Source: CAD feature listing. Evaluate the final solid. Frame: model axes, mm. Face numbers are marked on the shaded views. A direction names the side the tool comes from. Round coordinates to 2 decimals unless told otherwise and drop trailing zeros. Loops run counter-clockwise (first coordinate to the right, second up) from the corner with the lowest first, then second, coordinate; pieces in that order, holes last. Notation, with made-up numbers: (86.25, 60) -> (124.25, 60) arc R22 ccw to (124.25, 72) -> close; hole circle Ø11 at (-13, -39). An arc over 180 degrees is marked (long way). Put each result on its own line as item: value. Start each with the question number.
1. Cut plane D-D (z = 1.5). Return the cut outline in (x, y), then the cut area to 3 significant figures.
2. Cut plane B-B (y = 6.5). Return the cut outline in (x, z).
3. Contact query for flat-ended pins moving along their axis: pin 1 (1.5 mm diameter, centred on x = -18, y = 3.5, fed in from +Z); pin 2 (5.5 mm diameter, centred on y = 12, z = 8.5, fed in from -X); pin 3 (3 mm diameter, centred on x = -7, y = 14.5, fed in from +Z); pin 4 (5 mm diameter, centred on x = -7, y = 8.5, fed in from +Z). Output: stop coordinate, or through.
4. Material intervals for L1, parallel to Y at x = -1.25, z = 17.75; L2, parallel to Z at x = -3.5, y = 13.75; L3, parallel to Z at x = -16.5, y = 12, sorted ascending.
5. Set-up query: the marked faces 1, 2, 3, 4 and 5. Return all of +Z, -Z, +X, -X, +Y, -Y with unobstructed straight access to the full face (end or side cutting, diameter ignored); none if empty.
6. Cut plane C-C (z = 3.5). Return the cut outline in (x, y).
7. Cut plane A-A (x = -16). Return the cut outline in (y, z), then the cut area to 4 significant figures.
```python
from build123d import *

# Parameters (mm, degrees)
BOSS_EXTRUDE1_DEPTH = 20
CUT_EXTRUDE5_DEPTH  = 30
BOSS_EXTRUDE5_DEPTH = 20
CUT_EXTRUDE9_DEPTH  = 22
CUT_EXTRUDE10_DEPTH = 22
BOSS_EXTRUDE6_DEPTH = 5
BOSS_EXTRUDE7_DEPTH = 5
BOSS_EXTRUDE8_DEPTH = 5
CUT_EXTRUDE11_DEPTH = 5


with BuildPart() as part:
    # Sketch1 → Boss-Extrude1 (new body)
    with BuildSketch(Plane(origin=(0, 0, 0), x_dir=(1, 0, 0), z_dir=(0, 1, 0))):
        Polygon((-15, 0), (0, 0), (0, -15), (-5, -15), (-5, -10), align=None)
    extrude(amount=BOSS_EXTRUDE1_DEPTH)

    # Sketch8 → Cut-Extrude5 (cut)
    with BuildSketch(Plane.ZY.offset(5)):
        Polygon((10, 20), (15, 15), (15, 20), align=None)
    extrude(amount=-CUT_EXTRUDE5_DEPTH, mode=Mode.SUBTRACT)

    # Sketch9 → Boss-Extrude5 (add)
    with BuildSketch(Plane(origin=(0, 0, 0), x_dir=(-1, 0, 0), z_dir=(0, -1, 0))):
        Polygon((15, 0), (5, -10), (5, -15), (15, -15), align=None)
    extrude(amount=-BOSS_EXTRUDE5_DEPTH)

    # 3DSketch3 → Cut-Extrude9 (cut, along a direction that is not the sketch's normal)
    with BuildSketch(Plane(origin=(-15, 20, 0), x_dir=(0.2672612419124245, -0.5345224838248489, 0.8017837257372732), z_dir=(-0.5773502691896256, 0.5773502691896258, 0.5773502691896258))):
        Polygon((0, 0), (10.690449676, 9.258200998), (17.371980724, 6.943650748), (18.708286934, 0), (13.363062096, -4.629100499), align=None)
    extrude(amount=CUT_EXTRUDE9_DEPTH, dir=(0, 0, 1), mode=Mode.SUBTRACT)

    # Sketch11 → Cut-Extrude10 (cut)
    with BuildSketch(Plane(origin=(0, 10, 0), x_dir=(1, 0, 0), z_dir=(0, 1, 0))):
        Polygon((-15, -10), (-10, -15), (-15, -15), align=None)
    extrude(amount=-CUT_EXTRUDE10_DEPTH, mode=Mode.SUBTRACT)

    # Sketch12 → Boss-Extrude6 (add)
    with BuildSketch(Plane.XY.offset(15)):
        Polygon((-5, 10), (0, 10), (0, 0), (-10, 0), (-10, 5), align=None)
    extrude(amount=BOSS_EXTRUDE6_DEPTH)

    # Sketch13 → Boss-Extrude7 (add)
    with BuildSketch(Plane.ZY.offset(15)):
        Polygon((0, 0), (0, 15), (5, 15), (5, 10), (10, 5), (10, 0), align=None)
    extrude(amount=BOSS_EXTRUDE7_DEPTH)

    # Sketch14 → Boss-Extrude8 (add)
    with BuildSketch(Plane(origin=(0, 0, 0), x_dir=(-1, 0, 0), z_dir=(0, -1, 0))):
        Polygon((20, -10), (15, -10), (10, -15), (20, -15), align=None)
    extrude(amount=-BOSS_EXTRUDE8_DEPTH)

    # Sketch15 → Cut-Extrude11 (cut)
    with BuildSketch(Plane.XY.offset(15)):
        Polygon((-20, 0), (-20, 5), (-15, 5), align=None)
    extrude(amount=-CUT_EXTRUDE11_DEPTH, mode=Mode.SUBTRACT)


solid = part.part
```
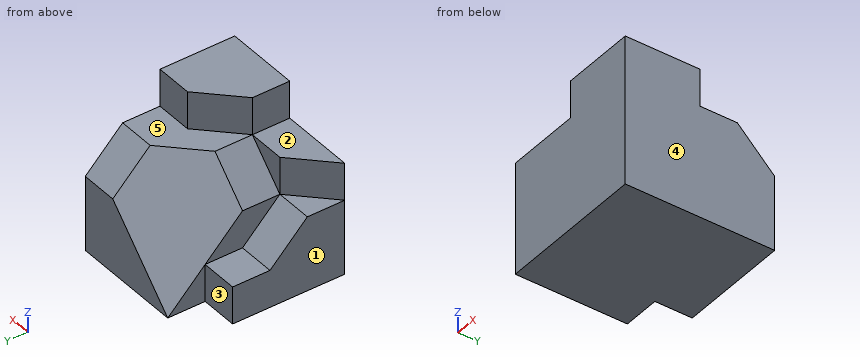
Solution:
1. outline: (-20, 0) -> (0, 0) -> (0, 20) -> (-13.5, 20) -> (-15, 18.5) -> (-15, 15) -> (-20, 15) -> close
1. area: 374 mm^2
2. outline: (-20, 0) -> (0, 0) -> (0, 20) -> (-8.5, 20) -> (-8.5, 15) -> (-10, 15) -> (-15, 10) -> (-15, 8.5) -> (-20, 8.5) -> close
3. pin 1: stops at z = 10
3. pin 2: stops at x = -15
3. pin 3: stops at z = 15
3. pin 4: stops at z = 20
4. L1: y = 0 to 10
4. L2: z = 0 to 15
4. L3: z = 0 to 5
5. face 1: +Z, -Z, -X, +Y, -Y
5. face 2: +Z, -X, +Y, -Y
5. face 3: +Z, -Z, -X, +Y
5. face 4: +Z, -Z, +X, +Y, -Y
5. face 5: +Z, -X, +Y
6. outline: (-20, 0) -> (0, 0) -> (0, 20) -> (-11.5, 20) -> (-15, 16.5) -> (-15, 15) -> (-20, 15) -> close
7. outline: (0, 0) -> (15, 0) -> (15, 5) -> (10, 5) -> (5, 10) -> (4, 10) -> (4, 15) -> (0, 15) -> close
7. area: 132.5 mm^2
